Autodesk Inventor part; units mm, degrees
ref_plane "YZ Plane" through (0, 0, 0) normal (1, 0, 0) x (0, 1, 0)
ref_plane "XZ Plane" through (0, 0, 0) normal (0, 1, 0) x (-1, 0, 0)
ref_plane "XY Plane" through (0, 0, 0) normal (0, 0, 1) x (1, 0, 0)
sketch "スケッチ2" plane through (0, 0, 0) normal (0, 0, 1) x (1, 0, 0)
  circle A0 centre (0, 0) radius 1.35
  line L0 (2.5, 0) -> (2.5, -56)
  circle A1 centre (0, 0) radius 2.4
  arc A2 (2.5, 0) -> (0, 2.4) centre (-0.046276, -0.150287) ccw
  arc A3 (0, 2.4) -> (-2.4, 0) centre (0, 0) ccw
  circle A4 centre (0, -27) radius 1.35
  circle A5 centre (-27, -27) radius 1.35
  line L1 (-7.25, -59) -> (2.5, -56)
  line L2 (-19.75, -56) -> (-19.75, -59)
  line L3 (-19.75, -59) -> (-29.5, -56)
  line L4 (-19.75, -59) -> (-7.25, -59)
  line L5 (-29.5, -56) -> (-29.5, -27)
  circle A6 centre (-8.3, -56) radius 1.05
  circle A7 centre (-8.3, -51) radius 1.05
  circle A8 centre (-18.7, -51) radius 1.05
  circle A9 centre (-18.7, -56) radius 1.05
  circle A10 centre (-2.75, -53.5) radius 1.55
  circle A11 centre (-24.25, -53.5) radius 1.55
  line L6 (-6.75, -48) -> (-20.25, -48)
  line L7 (-29.5, -27) -> (-27, -27)
  line L8 (-27, -27) -> (-28.554237, -25.041851)
  circle A12 centre (-27, -27) radius 2.5
  line L9 (-24.25, -44) -> (-24.25, -30.090988)
  line L10 (-2.75, -44) -> (-2.75, -18.930071)
  line L11 (-8.354493, -16.133446) -> (-22.655135, -26.894845)
  arc A13 (-28.554237, -25.041851) -> (-29.5, -27) centre (-27, -27) ccw
  line L12 (-28.554237, -25.041851) -> (-6.048598, -8.106096)
  arc A14 (-6.048598, -8.106096) -> (-2.4, 0) centre (-13.536142, 0.138263) ccw
  line L13 (-7.25, -56) -> (-7.25, -59)
  line L14 (-19.75, -56) -> (-7.25, -56)
  line L15 (-7.25, -56) -> (-7.25, -51)
  line L16 (-7.25, -51) -> (-19.75, -51)
  line L17 (-19.75, -51) -> (-19.75, -56)
  line L18 (-19.8, -50.95) -> (-7.2, -50.95)
  line L19 (-7.2, -50.95) -> (-7.2, -56.05)
  line L20 (-7.2, -56.05) -> (-19.8, -56.05)
  line L21 (-19.8, -56.05) -> (-19.8, -50.95)
  circle A15 centre (-18.7, -51) radius 1.1
  circle A16 centre (-8.3, -51) radius 1.1
  circle A17 centre (-18.7, -56) radius 1.1
  circle A18 centre (-8.3, -56) radius 1.1
  line L22 (2.5, -56) -> (-29.5, -56)
  circle A19 centre (-16, 1) radius 10.5
  arc A20 (-22.655135, -26.894845) -> (-24.25, -30.090988) centre (-20.25, -30.090988) ccw
  arc A21 (-24.25, -44) -> (-20.25, -48) centre (-20.25, -44) ccw
  arc A22 (-6.75, -48) -> (-2.75, -44) centre (-6.75, -44) ccw
  arc A23 (-2.75, -18.930071) -> (-8.354493, -16.133446) centre (-6.25, -18.930071) ccw
  point P0 (-2.75, -48)
  point P1 (-24.25, -48)
  point P2 (-24.25, -28.095)
  point P3 (-2.75, -11.916)
  point P4 (-19.798863, -50.95)
  point P5 (-17.601137, -50.95)
  point P6 (-9.398863, -50.95)
  point P7 (-7.201137, -50.95)
  point P8 (-7.201137, -56.05)
  point P9 (-9.398863, -56.05)
  point P10 (-17.601137, -56.05)
  point P11 (-19.798863, -56.05)
  dimension "d0" = 2.7
  dimension "d1" = 56
  dimension "d2" = 32
  dimension "d3" = 4.8
  dimension "d6" = 2.7
  dimension "d7" = 2.7
  dimension "d10" = 29
  dimension "d11" = 5
  dimension "d13" = 3.1
  dimension "d14" = 2.5
  dimension "d15" = 51.56
  dimension "d18" = 28.166
  dimension "d23" = 0.05
  dimension "d25" = 0.05
  dimension "d27" = 0.05
  dimension "d29" = 0.05
  dimension "d34" = 21
  dimension "d35" = 4
  dimension "d36" = 3.5
sketch "スケッチ2 outline for 押し出し2" plane through (0, 0, 0) normal (0, 0, 1) x (1, 0, 0)
  line L0 (-29.5, -27) -> (-29.5, -56)
  arc A0 (-28.554237, -25.041851) -> (-29.5, -27) centre (-27, -27) ccw
  line L1 (-29.5, -56) -> (-19.75, -59)
  line L2 (-6.048598, -8.106096) -> (-28.554237, -25.041851)
  line L3 (-19.75, -59) -> (-7.25, -59)
  arc A1 (-2.4, 0) -> (-6.048598, -8.106096) centre (-13.536142, 0.138263) cw
  line L4 (-7.25, -59) -> (2.5, -56)
  arc A2 (0, 2.4) -> (-2.4, 0) centre (0, 0) ccw
  line L5 (2.5, -56) -> (2.5, 0)
  arc A3 (2.5, 0) -> (0, 2.4) centre (-0.046276, -0.150287) ccw
  circle A4 centre (-24.25, -53.5) radius 1.55
  line L6 (-6.75, -48) -> (-20.25, -48)
  arc A5 (-2.75, -44) -> (-6.75, -48) centre (-6.75, -44) cw
  line L7 (-2.75, -18.930071) -> (-2.75, -44)
  arc A6 (-8.354493, -16.133446) -> (-2.75, -18.930071) centre (-6.25, -18.930071) cw
  line L8 (-22.655135, -26.894845) -> (-8.354493, -16.133446)
  arc A7 (-24.25, -30.090988) -> (-22.655135, -26.894845) centre (-20.25, -30.090988) cw
  line L9 (-24.25, -44) -> (-24.25, -30.090988)
  arc A8 (-20.25, -48) -> (-24.25, -44) centre (-20.25, -44) cw
  line L10 (-19.798863, -56.05) -> (-19.8, -50.95)
  arc A9 (-17.601137, -56.05) -> (-19.798863, -56.05) centre (-18.7, -56) cw
  line L11 (-9.398863, -56.05) -> (-17.601137, -56.05)
  arc A10 (-7.2, -56.05) -> (-9.398863, -56.05) centre (-8.299432, -55.999405) cw
  line L12 (-7.201137, -50.95) -> (-7.2, -56.05)
  arc A11 (-9.398863, -50.95) -> (-7.201137, -50.95) centre (-8.3, -51) cw
  line L13 (-17.601137, -50.95) -> (-9.398863, -50.95)
  arc A12 (-19.8, -50.95) -> (-17.601137, -50.95) centre (-18.700568, -51.000595) cw
  circle A13 centre (-2.75, -53.5) radius 1.55
  circle A14 centre (-27, -27) radius 1.35
  circle A15 centre (0, -27) radius 1.35
  circle A16 centre (0, 0) radius 1.35
extrude "押し出し2" add sketch "スケッチ2 outline for 押し出し2" along normal blind 2
fillet "フィレット3" radius 4 4 edges at (-29.5, -56, 1) (-19.75, -59, 1) (-7.25, -59, 1) (2.5, -56, 1)
properties part number "UpperArm_vertical_frame_01"
The model under review builds one solid part; all positions refer to its coordinate system, in mm. A direction names the side the tool comes from. Coordinates: 2 decimals unless noted, no trailing zeros. Loops run counter-clockwise (first coordinate to the right, second up) from the corner with the lowest first, then second, coordinate; pieces in that order, holes last. Notation, with made-up numbers: (28, -1) -> (78, -1) arc R17 cw to (78, 27) -> close; hole circle Ø9 at (38.25, 2.5). An arc over 180 degrees is marked (long way). Use a Markdown table: item, result. Add a question column.
1. To check wall thickness, follow line 1 (X direction, y = -36, z = 1.15); line 2 (Y direction, x = 0, z = 1.35); line 3 (Y direction, x = -11.5, z = 1.7). State the ranges of each line that lie inside material, in increasing order.
2. Add section D-D on x = -3.5. Write out the cut boundary in (y, z) (3 decimals).
3. Add section B-B on x = -14.5. Write out the cut boundary in (y, z).
4. Add section A-A on y = -39. Write out the cut boundary in (x, z), plus the area to 3 significant figures.
5. Clearance check with a flat-ended pin moving along its axis: pin 1 Ø4 at (x, y) = (-2.75, -53.5) entering from +Z. State where the tip first meets the part, or that it passes through.
6. Machinability: for faces 1 (the face through (-29.5, -40, 1)), 2 (the face through (-24.25, -37, 1)), which of the approach directions +Z, -Z, +X, -X, +Y, -Y give a long, thin tool a straight path to every point of the face, cutting with its end or side? Answer none if there is none.
7. Add section C-C on z = 1.15. Give the number of separate pieces and of enclosed holes in the cut face, plus the area to 3 significant figures.
8. Draft analysis for pull direction X (two halves, no side actions). For faces 3 (the face through (-1.716, 1.678, 0.986)), 4 (the face through (-18.7, -57.1, 1)), 5 (the face through (-13.7, -48.3, 0)), state which applies: pulls with the +X half, pulls with the -X half, needs draft (parallel to the pull), parting line crosses it, or undercut.
Returned:
| question | item | result |
|---|---|---|
| 1 | line 1 | x = -29.5 to -24.25, -2.75 to 2.5 |
| 1 | line 2 | y = -56.75 to -28.35, -25.65 to -1.35, 1.35 to 2.4 |
| 1 | line 3 | y = -59 to -56.05, -50.95 to -48, -18.5 to -12.21 |
| 2 | outline | (-57.846, 0) -> (-54.856, 0) -> (-54.856, 2) -> (-57.846, 2) -> close; (-52.144, 0) -> (-46.332, 0) -> (-46.332, 2) -> (-52.144, 2) -> close; (-16.765, 0) -> (-4.69, 0) -> (-4.69, 2) -> (-16.765, 2) -> close |
| 3 | outline | (-59, 0) -> (-56.05, 0) -> (-56.05, 2) -> (-59, 2) -> close; (-50.95, 0) -> (-48, 0) -> (-48, 2) -> (-50.95, 2) -> close; (-20.76, 0) -> (-14.47, 0) -> (-14.47, 2) -> (-20.76, 2) -> close |
| 4 | outline | (-29.5, 0) -> (-24.25, 0) -> (-24.25, 2) -> (-29.5, 2) -> close; (-2.75, 0) -> (2.5, 0) -> (2.5, 2) -> (-2.75, 2) -> close |
| 4 | area | 21.0 mm² |
| 5 | pin 1 | stops at z = 2 |
| 6 | face 1 | +Z, -Z, -X, +Y, -Y |
| 6 | face 2 | +Z, -Z |
| 7 | separate pieces | 1 |
| 7 | enclosed holes | 7 |
| 7 | area | 760 mm² |
| 8 | face 3 | pulls with the -X half |
| 8 | face 4 | undercut |
| 8 | face 5 | needs draft |
